Autodesk Fusion 360 part; units mm, degrees
sketch "Sketch1" plane through (0, 0, 0) normal (0, 1, 0) x (1, 0, 0)
  line L0 (0, 0) -> (-58, 0)
  line L1 (-58, 0) -> (-58, -20)
  line L2 (-58, -20) -> (0, -20)
  line L3 (0, -20) -> (0, 0)
extrude "Extrude1" add sketch "Sketch1" against normal blind 2
sketch "Sketch2" plane through (0, 0, 0) normal (0, 1, 0) x (1, 0, 0)
  line L0 (-60, -22) -> (2, -22)
  line L1 (2, -22) -> (2, -20)
  line L2 (2, -20) -> (-60, -20)
  line L3 (-60, -20) -> (-60, -22)
extrude "Extrude2" add sketch "Sketch2" against normal blind 7
sketch "Sketch3" plane through (0, 0, 0) normal (0, 1, 0) x (1, 0, 0)
  line L0 (-60, 0) -> (2, 0)
  line L1 (2, 0) -> (2, 2)
  line L2 (2, 2) -> (-60, 2)
  line L3 (-60, 2) -> (-60, 0)
extrude "Extrude3" add sketch "Sketch3" against normal blind 7
sketch "Sketch4" plane through (0, 0, 0) normal (0, 1, 0) x (1, 0, 0)
  line L0 (0, -20) -> (2, -20)
  line L1 (2, -20) -> (2, 0)
  line L2 (2, 0) -> (0, 0)
  line L3 (0, 0) -> (0, -20)
extrude "Extrude4" add sketch "Sketch4" against normal blind 7
sketch "Sketch5" plane through (0, 0, 0) normal (0, 1, 0) x (1, 0, 0)
  line L0 (-42, -20) -> (-37, -20)
  line L1 (-37, -20) -> (-37, 0)
  line L2 (-37, 0) -> (-42, 0)
  line L3 (-42, 0) -> (-42, -20)
sketch "Sketch6" plane through (0, 0, 0) normal (0, 1, 0) x (1, 0, 0)
extrude "Extrude5" add sketch "Sketch5" against normal blind 5
sketch "Sketch7" plane through (0, 0, 0) normal (0, 1, 0) x (1, 0, 0)
  line L0 (-15, -20) -> (-20, -20)
  line L1 (-20, -20) -> (-20, 0)
  line L2 (-20, 0) -> (-15, 0)
  line L3 (-15, 0) -> (-15, -20)
extrude "Extrude6" add sketch "Sketch7" against normal blind 5
extrude "Extrude7" add 1 faces at (-60, -2.3333, 20.6667) along direction (-1, 0, 0) blind 5
extrude "Extrude8" add 1 faces at (-60, -2.3333, -1.3333) along direction (-1, 0, 0) blind 5
extrude "Extrude9" add 1 faces at (-21, -7, -1.3333) along direction (0, -1, 0) blind 18
sketch "Sketch8" plane through (0, 0, 0) normal (1, 0, 0) x (0, 1, 0)
  line L0 (-7, 5) -> (-11, 5)
  line L1 (-11, 5) -> (-11, 15)
  line L2 (-11, 15) -> (-7, 15)
  line L3 (-7, 15) -> (-7, 5)
extrude "Extrude10" cut sketch "Sketch8" along normal blind 2
sketch "Sketch9" plane through (0, 0, 0) normal (0, 1, 0) x (1, 0, 0)
  line L0 (-60, -20) -> (-58, -20)
  line L1 (-58, -20) -> (-58, 0)
  line L2 (-58, 0) -> (-60, 0)
  line L3 (-60, 0) -> (-60, -20)
  dimension "d21" = 2
extrude "Extrude11" add sketch "Sketch9" against normal blind 6
Verification items for the finished model (mm, model axes). A direction names the side the tool comes from. Round coordinates to 2 decimals unless told otherwise and drop trailing zeros. Order: outer loops, then holes, each group sorted by start corner. A loop starts at its lowest first (then second) coordinate and runs counter-clockwise, first axis right, second up. Notation, with made-up numbers: (35, 9) -> (62, 9) arc R19 ccw to (62, 34) -> close; hole circle Ø8 at (26.5, 27). An arc over 180 degrees is marked (long way). Put each result on its own line as item: value. Start each with the question number.
(1) Section check B-B (y = -2.75). Enter the section's corners in (x, z).
(2) Material ranges on line 1 along X through (y, z) = (-3.5, 3.75); line 2 along Z through (x, y) = (-62, -8); line 3 along X through (y, z) = (-17.5, 5.25), recorded low to high.
(3) Section check A-A (z = 11.75). Enter the section's corners in (x, y).
(4) Draft check along Y on faces 1 (the face through (-20, -3, 10)), 2 (the face through (1, -11, 10)), 3 (the face through (-40, -5, 10)). Enter one of: +Y half, -Y half, draft (parallel to the pull), parting line (faces both ways), or undercut.
(5) Depth check by flat-ended pin: pin 1 Ø1.5 at (y, z) = (-3, 12) entering from -X; pin 2 Ø8.5 at (x, z) = (-24.5, 9.5) entering from -Y; pin 3 Ø4 at (x, z) = (-17, 12) entering from -Y. Enter the tip coordinate at first touch or a pass-through.
(6) Section check C-C (y = -9). Enter the section's corners in (x, z), then the cut area to 3 significant figures.
(7) Tool access check on faces 4 (the face through (-15, -3, 10)), 5 (the face through (-60, -3, 10)), 6 (the face through (1, -9, 5)). Record the directions out of +Z, -Z, +X, -X, +Y, -Y that give a thin tool (end or side, any length) a straight path to the whole face; none if there is none.
(8) Section check D-D (z = 17.25). Enter the section's corners in (x, y), then the cut area to 3 significant figures.
Completed:
1. outline: (-65, -2) -> (2, -2) -> (2, 22) -> (-65, 22) -> (-65, 20) -> (-60, 20) -> (-60, 0) -> (-65, 0) -> close; hole (-58, 0) -> (-42, 0) -> (-42, 20) -> (-58, 20) -> close; hole (-37, 0) -> (-20, 0) -> (-20, 20) -> (-37, 20) -> close; hole (-15, 0) -> (0, 0) -> (0, 20) -> (-15, 20) -> close
2. line 1: x = -60 to -58, -42 to -37, -20 to -15, 0 to 2
2. line 2: z = -2 to 0, 20 to 22
2. line 3: x = 0 to 2
3. outline: (-60, -6) -> (-58, -6) -> (-58, -2) -> (-42, -2) -> (-42, -5) -> (-37, -5) -> (-37, -2) -> (-20, -2) -> (-20, -5) -> (-15, -5) -> (-15, -2) -> (0, -2) -> (0, -7) -> (2, -7) -> (2, 0) -> (-60, 0) -> close; (0, -25) -> (2, -25) -> (2, -11) -> (0, -11) -> close
4. face 1: draft
4. face 2: undercut
4. face 3: -Y half
5. pin 1: stops at x = -60
5. pin 2: stops at y = -2
5. pin 3: stops at y = -5
6. outline: (-65, -2) -> (2, -2) -> (2, 5) -> (0, 5) -> (0, 0) -> (-65, 0) -> close; (-65, 20) -> (0, 20) -> (0, 15) -> (2, 15) -> (2, 22) -> (-65, 22) -> close
6. area: 288 mm2
7. face 4: -Y
7. face 5: -X, +Y, -Y
7. face 6: +X, -X
8. outline: (-60, -6) -> (-58, -6) -> (-58, -2) -> (-42, -2) -> (-42, -5) -> (-37, -5) -> (-37, -2) -> (-20, -2) -> (-20, -5) -> (-15, -5) -> (-15, -2) -> (0, -2) -> (0, -25) -> (2, -25) -> (2, 0) -> (-60, 0) -> close
8. area: 208 mm2
